Job drawing, mm, ordinate dimensions from the low corner. One solid piece. Give positions to 0.01 mm unless a question says otherwise; leave off trailing zeros. Write each loop counter-clockwise with the first axis right and the second up, starting at its lowest first coordinate (ties: lowest second). Pieces come first, ordered by that corner, then holes. Notation, with made-up numbers: M 49.5,73.25 L 78.5,73.25 A23 ccw 78.5,89.25 Z; hole C 17.5,50 d11. An arc over 180 degrees is marked long. Answer as CSV lines item,"result". Start each with the question number.
Item 1: Wall check: L1, parallel to Z at x = 39.5, y = 2.15; L2, parallel to Z at x = 96.5, y = 2.5; L3, parallel to X at y = 0.75, z = 110.5. Give the ranges that are in metal, low to high. Write a range as from..to.
Item 2: Pin check, flat tip, straight feed: pin 1 (19.5 mm diameter, centred on x = 39.5, z = 50, fed in from +Y). Stop position of the tip, or through.
Item 3: Band-saw the part on A-A, the plane x = 99.5. List the corners of the cut face in (y, z), then the cut area to 3 significant figures.
Item 4: Band-saw the part on D-D, the plane x = 24.5. List the corners of the cut face in (y, z), then the cut area to 3 significant figures.
Item 5: Band-saw the part on B-B, the plane y = 1.9. Count the separate pieces of the cut face and the enclosed holes in it, then the cut area to 3 significant figures.
Item 6: Band-saw the part on C-C, the plane z = 80. List the corners of the cut face in (x, y).
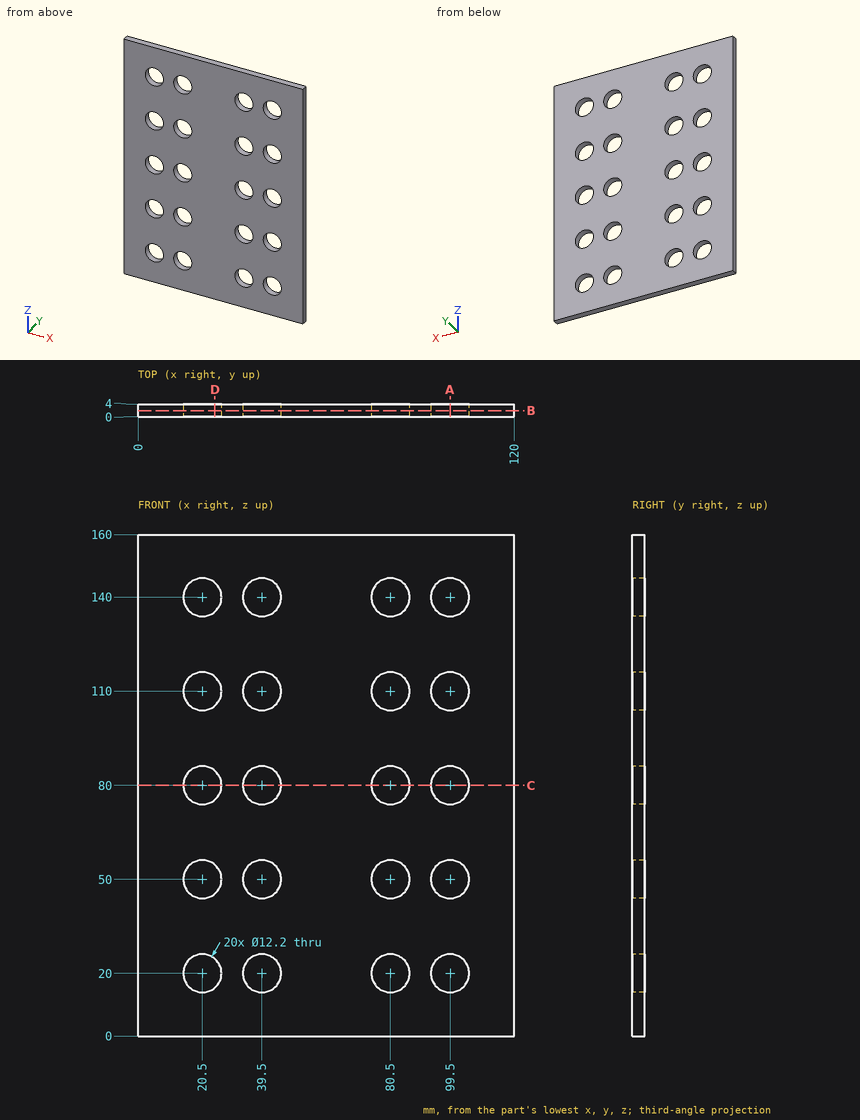
Output:
1,L1,"0..13.9, 26.1..43.9, 56.1..73.9, 86.1..103.9, 116.1..133.9, 146.1..160"
1,L2,"0..14.69, 25.31..44.69, 55.31..74.69, 85.31..104.69, 115.31..134.69, 145.31..160"
1,L3,"0..14.42, 26.58..33.42, 45.58..74.42, 86.58..93.42, 105.58..120"
2,pin 1,"y = 4"
3,outline,"M 0,0 L 4,0 L 4,13.9 L 0,13.9 Z; M 0,26.1 L 4,26.1 L 4,43.9 L 0,43.9 Z; M 0,56.1 L 4,56.1 L 4,73.9 L 0,73.9 Z; M 0,86.1 L 4,86.1 L 4,103.9 L 0,103.9 Z; M 0,116.1 L 4,116.1 L 4,133.9 L 0,133.9 Z; M 0,146.1 L 4,146.1 L 4,160 L 0,160 Z"
3,area,"396 mm²"
4,outline,"M 0,0 L 4,0 L 4,15.39 L 0,15.39 Z; M 0,24.61 L 4,24.61 L 4,45.39 L 0,45.39 Z; M 0,54.61 L 4,54.61 L 4,75.39 L 0,75.39 Z; M 0,84.61 L 4,84.61 L 4,105.39 L 0,105.39 Z; M 0,114.61 L 4,114.61 L 4,135.39 L 0,135.39 Z; M 0,144.61 L 4,144.61 L 4,160 L 0,160 Z"
4,area,"456 mm²"
5,separate pieces,"1"
5,enclosed holes,"20"
5,area,"16,900 mm²"
6,outline,"M 0,0 L 14.4,0 L 14.4,4 L 0,4 Z; M 26.6,0 L 33.4,0 L 33.4,4 L 26.6,4 Z; M 45.6,0 L 74.4,0 L 74.4,4 L 45.6,4 Z; M 86.6,0 L 93.4,0 L 93.4,4 L 86.6,4 Z; M 105.6,0 L 120,0 L 120,4 L 105.6,4 Z"
